Autodesk Inventor part; units mm, degrees
ref_plane "YZ Plane" through (0, 0, 0) normal (1, 0, 0) x (0, 1, 0)
ref_plane "XZ Plane" through (0, 0, 0) normal (0, 1, 0) x (-1, 0, 0)
ref_plane "XY Plane" through (0, 0, 0) normal (0, 0, 1) x (1, 0, 0)
sketch "Sketch1" plane through (0, 0, 0) normal (1, 0, 0) x (0, 1, 0)
  line L0 (0, 0) -> (0, 8.5)
  line L1 (0, 14.5) -> (6, 14.5)
  line L2 (0, 0) -> (0, -8.5)
  line L3 (0, -14.5) -> (6, -14.5)
  line L4 (6, -14.5) -> (6, -8.5)
  line L5 (6, -8.5) -> (0, -8.5)
  line L6 (6, 14.5) -> (6, 8.5)
  line L7 (6, 8.5) -> (0, 8.5)
  line L8 (0, 14.5) -> (-3, 14.5)
  line L9 (-3, 14.5) -> (-3, -14.5)
  line L10 (-3, -14.5) -> (0, -14.5)
  line L11 (0, -8.5) -> (-3, -8.5)
  line L12 (0, 8.5) -> (-3, 8.5)
  line L13 (-3, 0) -> (-3, -5)
  dimension "d0" = 14.5
  dimension "d1" = 6
  dimension "d2" = 14.5
  dimension "d3" = 6
  dimension "d4" = 90
  dimension "d5" = 29
  dimension "d6" = 6
  dimension "d7" = 6
  dimension "d8" = 3
  dimension "d9" = 5
extrude "Extrusion1" add sketch "Sketch1" along normal mid plane 5
sketch "Sketch2" plane through (2.5, 0, 0) normal (1, 0, 0) x (0, 0, -1)
  line L0 (8.5, 0) -> (-8.5, 0)
  line L1 (0, 0) -> (-8.5, 0)
  line L2 (-8.5, 0) -> (-11.5, 0)
  line L3 (-14.5, 6) -> (-14.5, -3)
  line L4 (-11.5, 0) -> (-11.5, 3)
  line L5 (8.5, 0) -> (11.5, 0)
  line L6 (11.5, 0) -> (11.5, 3)
  circle A0 centre (-11.5, 3) radius 1.5
  circle A1 centre (11.5, 3) radius 1.5
  dimension "d14" = 3
  dimension "d15" = 3
  dimension "d16" = 3
  dimension "d17" = 3
  dimension "d18" = 3
  dimension "d19" = 3
extrude "Extrusion2" cut sketch "Sketch2" against normal blind 10
sketch "Sketch3" plane through (-2.5, 0, 0) normal (-1, 0, 0) x (0, 0, 1)
  circle A0 centre (-11.5, 3) radius 1.5
  circle A1 centre (-11.5, 3) radius 3
  line L0 (-14.5, 3) -> (-14.5, 7.7039)
  line L1 (-14.5, -3) -> (-14.5, 6)
  line L2 (-14.5, 7.7039) -> (-8.5, 7.7039)
  line L3 (-8.5, 7.7039) -> (-8.5, 3)
  circle A2 centre (11.5, 3) radius 1.5
  circle A3 centre (11.5, 3) radius 3
  line L4 (8.5, 3) -> (8.5, 6.9796)
  line L5 (8.5, 6.9796) -> (14.5, 6.9796)
  line L6 (14.5, 6.9796) -> (14.5, 3)
  line L7 (14.5, 6) -> (14.5, -3)
  point P0 (0, 0)
extrude "Extrusion3" cut sketch "Sketch3" against normal through all contours A1 L0 L2 L3 | A3 L4 L5 L6
sketch "Sketch4" plane through (2.5, 0, 0) normal (1, 0, 0) x (0, 0, -1)
  line L0 (14.5, -3) -> (-14.5, -3)
  line L1 (0, -3) -> (4, -3)
  line L2 (0, -3) -> (-4, -3)
  line L3 (-4, -3) -> (-4, -1.5)
  line L4 (-4, -1.5) -> (4, -1.5)
  line L5 (4, -1.5) -> (4, -6.5)
  line L6 (4, -6.5) -> (-4, -6.5)
  line L7 (-4, -6.5) -> (-4, -1.5)
  point P0 (0, 0)
  dimension "d24" = 4
  dimension "d25" = 4
  dimension "d26" = 1.5
  dimension "d27" = 5
  dimension "d28" = 8
extrude "Extrusion4" add sketch "Sketch4" against normal blind 10
sketch "Sketch24" plane through (-7.5, -1.5, -4) normal (0, 1, 0) x (1, 0, 0)
  line L0 (0, -8) -> (0, 0)
  line L1 (0, 0) -> (0, -4)
  line L2 (5, -8) -> (0, -8)
  line L3 (0, -4) -> (0, -5.075)
  line L4 (0, -4) -> (0, -2.925)
  line L5 (0, -4) -> (-2.65, -4)
  line L6 (-2.65, -4) -> (-2.65, -6.075)
  line L7 (-2.65, -4) -> (-0.575, -4) construction
  line L8 (-2.65, -4) -> (-2.65, -1.925)
  line L9 (-2.65, -1.925) -> (0, -2.925)
  line L10 (0, -5.075) -> (-2.65, -6.075)
  point P0 (7.5, -4)
  dimension "d150" = 4
  dimension "d151" = 1.075
  dimension "d152" = 1.075
  dimension "d153" = 2.65
  dimension "d154" = 2.075
  dimension "d155" = 90
  dimension "d156" = 2.075
extrude "Extrusion20" add sketch "Sketch24" along normal mid plane 15
sketch "Sketch25" plane through (2.5, -6.5, -4) normal (0, -1, 0) x (1, 0, 0)
  line L0 (-10, 2.925) -> (-12.65, 1.925)
  line L1 (-12.65, 1.925) -> (-12.65, 6.075)
  line L2 (-12.65, 1.925) -> (-12.65, 6.075)
  line L3 (-10, 8) -> (-10, 5.075)
  line L4 (-12.65, 6.075) -> (-10, 5.075)
  line L5 (-10, 5.075) -> (-10, 2.925)
  line L6 (-10, 5.075) -> (-10, 2.925)
  line L7 (-10, 2.925) -> (-12.65, 1.925)
  point P0 (-2.5, 4)
extrude "Extrusion21" add sketch "Sketch25" along normal blind 7.5
properties part number "pelvis øvre del"
Build history of the part. All positions in model axes, mm. A direction names the side the tool comes from. Round coordinates to 2 decimals unless told otherwise and drop trailing zeros. Write each loop counter-clockwise with the first axis right and the second up, starting at its lowest first coordinate (ties: lowest second). Pieces come first, ordered by that corner, then holes. Notation, with made-up numbers: (-18.75, 20.5) - (5.25, 20.5) arc R16 ccw to (5.25, 30.5) - close; hole circle Ø10 at (-27, 15). An arc over 180 degrees is marked (long way). One line per question, with ' | ' between items.
1. Drop flat-ended pins along their axis: pin 1 Ø3 at (x, y) = (0.5, -5) entering from +Z; pin 2 Ø1.7 at (y, z) = (2.5, -0.5) entering from +X; pin 3 Ø5 at (x, y) = (-8, -8) entering from -Z; pin 4 Ø5 at (y, z) = (3, 11.5) entering from +X. Give the stop position or say it passes through.
Results are:
pin 1: z = 4 | pin 2: x = -7.5 | pin 3: z = -4 | pin 4: x = 2.5
2. Band-saw the part on C-C, the plane y = -6. Write the cut outline in (x, z) (3 decimals), and give its area (3 significant figures).
Results are:
outline: (-10.15, -2.075) - (-7.5, -1.075) - (-7.5, -4) - (2.5, -4) - (2.5, 4) - (-7.5, 4) - (-7.5, 1.075) - (-10.15, 2.075) - close | area: 88.3 mm^2
3. Tool access for faces 4 (the face through (-8.84, -3.86, 1.58)), 5 (the face through (-2, -6.5, 0)), 6 (the face through (-7.5, -4, -3)): list every direction of +Z, -Z, +X, -X, +Y, -Y with a clear straight run to the whole face (end or side of a thin tool).
Results are:
face 4: +Z, +Y, -Y | face 5: +Z, -Z, +X, -Y | face 6: -Z, +Y, -Y
4. Band-saw the part on A-A, the plane z = -11.5. Write the cut outline in (x, y), and give its area (3 significant figures).
Results are:
outline: (-2.5, -3) - (2.5, -3) - (2.5, 1.5) - (-2.5, 1.5) - close; (-2.5, 4.5) - (2.5, 4.5) - (2.5, 6) - (-2.5, 6) - close | area: 30.0 mm^2
5. Band-saw the part on B-B, the plane x = 0.25. Write the cut outline in (y, z).
Results are:
outline: (-6.5, -4) - (-3, -4) - (-3, -14.5) - (3, -14.5) arc R3 ccw to (3, -8.5) - (0, -8.5) - (0, 8.5) - (3, 8.5) arc R3 ccw to (3, 14.5) - (-3, 14.5) - (-3, 4) - (-6.5, 4) - close; hole circle Ø3 at (3, -11.5); hole circle Ø3 at (3, 11.5)
6. Mould opens along Y. For faces 1 (the face through (0, 2.1, 12.7)), 2 (the face through (0, 0, 0)), 3 (the face through (-7.5, 2, 0)) say: released by +Y, released by -Y, zero draft, split by the parting line, or undercut.
Results are:
face 1: undercut | face 2: released by +Y | face 3: zero draft
7. Drill centre lines: line 1 along Z through (x, y) = (-1.3, 3); line 2 along Z through (x, y) = (-0.75, 3.75); line 3 along Y through (x, z) = (-2, 8). Where is each one in solid material? Low to high. Write a range as from..to.
Results are:
line 1: -14.5..-13, -10..-8.5, 8.5..10, 13..14.5 | line 2: -14.4..-12.8, -10.2..-8.6, 8.6..10.2, 12.8..14.4 | line 3: -3..0
8. Band-saw the part on D-D, the plane z = -1.75. Write the cut outline in (x, y).
Results are:
outline: (-10.15, -14) - (-9.29, -14) - (-9.29, 6) - (-10.15, 6) - close; (-7.5, -6.5) - (2.5, -6.5) - (2.5, 0) - (-2.5, 0) - (-2.5, -1.5) - (-7.5, -1.5) - close
